The listing builds one solid part. Answer for the finished solid, in the listing's coordinates (mm). Coordinates: 2 decimals unless noted, no trailing zeros. Write each loop counter-clockwise with the first axis right and the second up, starting at its lowest first coordinate (ties: lowest second). Pieces come first, ordered by that corner, then holes.
from build123d import *

# Parameters (mm, degrees)
SKETCH1_W           = 203.2
SKETCH1_H           = 203.2
BASE_FLANGE1_DEPTH  = 1.5875
SKETCH6_R           = 1.5875
SKETCH6_R_2         = 2.413
SKETCH6_R_3         = 9.525
CUT_EXTRUDE1_DEPTH  = 288.372580731
BREAK_CORNER1_START = -1.5875
BREAK_CORNER1_DEPTH = 1.5875
SKETCH7_R           = 6.985
SKETCH7_R_2         = 13.97
SKETCH7_R_3         = 7.9375
SKETCH7_R_4         = 3.175
SKETCH7_R_5         = 2.159
CUT_EXTRUDE2_DEPTH  = 288.372580731


# Read off the part's stored shape, not the designer's step: Break-Corner1
# Sheet-metal steps are written as plain solids
with BuildPart() as part:
    # Sketch1 → Base-Flange1 (new body)
    with BuildSketch(Plane.XY):
        with Locations((101.6, 101.6)):
            Rectangle(SKETCH1_W, SKETCH1_H)
    extrude(amount=-BASE_FLANGE1_DEPTH)

    # Sketch6 → Cut-Extrude1 (cut, through all)
    with BuildSketch(Plane(origin=(0, 0, -1.5875), x_dir=(-1, 0, 0), z_dir=(0, 0, -1))):
        with Locations((-19.05, 139.7)):
            Circle(SKETCH6_R)
        with Locations((-19.05, 12.7)):
            Circle(SKETCH6_R)
        with Locations((-31.115, 48.768)):
            Circle(SKETCH6_R_2)
        with Locations((-31.115, 12.7)):
            Circle(SKETCH6_R_2)
        with Locations((-172.085, 48.768)):
            Circle(SKETCH6_R_2)
        with Locations((-172.085, 12.7)):
            Circle(SKETCH6_R_2)
        with Locations((-184.15, 139.7)):
            Circle(SKETCH6_R)
        with Locations((-184.15, 12.7)):
            Circle(SKETCH6_R)
        with Locations((-190.5, 38.1)):
            Circle(SKETCH6_R_3)
        with Locations((-190.5, 114.3)):
            Circle(SKETCH6_R_3)
        with Locations((-12.7, 114.3)):
            Circle(SKETCH6_R_3)
        with Locations((-12.7, 38.1)):
            Circle(SKETCH6_R_3)
        with Locations((-6.35, 76.2)):
            Circle(SKETCH6_R)
        with Locations((-196.85, 76.2)):
            Circle(SKETCH6_R)
    extrude(amount=-CUT_EXTRUDE1_DEPTH, mode=Mode.SUBTRACT)

    # Break-Corner1 outline → Break-Corner1 (cut)
    with BuildSketch(Plane.XY.offset(BREAK_CORNER1_START)):
        Polygon((0, 0), (3.175, 0), (0, 3.175), align=None)
        Polygon((203.2, 3.175), (200.025, 0), (203.2, 0), align=None)
        Polygon((0, 203.2), (0, 200.025), (3.175, 203.2), align=None)
        Polygon((200.025, 203.2), (203.2, 200.025), (203.2, 203.2), align=None)
    extrude(amount=BREAK_CORNER1_DEPTH, mode=Mode.SUBTRACT)

    # Sketch7 → Cut-Extrude2 (cut, through all)
    with BuildSketch(Plane(origin=(0, 0, -1.5875), x_dir=(-1, 0, 0), z_dir=(0, 0, -1))):
        with Locations((-177.8, 177.8)):
            Circle(SKETCH7_R)
        with Locations((-101.6, 177.8)):
            Circle(SKETCH7_R_2)
        with Locations((-25.4, 177.8)):
            Circle(SKETCH7_R)
        with Locations((-101.6, 114.3)):
            Circle(SKETCH7_R_3)
        with Locations((-112.7125, 93.218)):
            Circle(SKETCH7_R_4)
        with Locations((-90.4875, 93.218)):
            Circle(SKETCH7_R_4)
        with Locations((-130.556, 85.09)):
            Circle(SKETCH7_R_5)
        with Locations((-73.66, 67.31)):
            Circle(SKETCH7_R_5)
    extrude(amount=-CUT_EXTRUDE2_DEPTH, mode=Mode.SUBTRACT)


solid = part.part
1. Section C-C on z = -0.8 is taken. State how many separate pieces and enclosed holes the cut face has, then the cut area to 3 significant figures.
Results found:
separate pieces: 1
enclosed holes: 22
area: 38,800 mm2
2. Flat-ended cylindrical pins translate along their axes: P1, Ø10, axis at x = 24.5, y = 65.5, coming from the +Z side; P2, Ø3.5, axis at x = 130.556, y = 85.09, coming from the +Z side. Find the tip coordinate at first contact, or state that the pin passes through.
Results found:
P1: stops at z = 0
P2: passes through
3. Section B-B on y = 177.8 is taken. Give the vertices of the cut face in (x, z) (1 decimal).
Results found:
outline: (0, -1.6) - (18.4, -1.6) - (18.4, 0) - (0, 0) - close; (32.4, -1.6) - (87.6, -1.6) - (87.6, 0) - (32.4, 0) - close; (115.6, -1.6) - (170.8, -1.6) - (170.8, 0) - (115.6, 0) - close; (184.8, -1.6) - (203.2, -1.6) - (203.2, 0) - (184.8, 0) - close
4. Find the intervals of material crossed by L1, parallel to X at y = 139.7, z = -0.7; L2, parallel to Y at x = 190.5, z = -1.4 (3 decimals); L3, parallel to Y at x = 19.05, z = -0.7, in increasing order.
Results found:
L1: x = 0 to 17.46, 20.64 to 182.56, 185.74 to 203.2
L2: y = 0 to 28.575, 47.625 to 104.775, 123.825 to 203.2
L3: y = 0 to 11.11, 14.29 to 31, 45.2 to 107.2, 121.4 to 138.11, 141.29 to 174.89, 180.71 to 203.2
5. For a pull along X with two mould halves and no side action, classify faces 1 (the cylindrical face through (19.72, 120.74, -0.8)), 2 (the flat face through (100, 103, -1.588)) as pulls with the +X half, pulls with the -X half, needs draft (parallel to the pull), parting line crosses it, or undercut.
Results found:
face 1: undercut
face 2: needs draft
6. Section A-A on x = 25.4 is taken. Give the vertices of the cut face in (y, z) (1 decimal).
Results found:
outline: (0, -1.6) - (170.8, -1.6) - (170.8, 0) - (0, 0) - close; (184.8, -1.6) - (203.2, -1.6) - (203.2, 0) - (184.8, 0) - close
7. Section D-D on x = 112.5 is taken. Give the vertices of the cut face in (y, z).
Results found:
outline: (0, -1.59) - (90.05, -1.59) - (90.05, 0) - (0, 0) - close; (96.39, -1.59) - (169.06, -1.59) - (169.06, 0) - (96.39, 0) - close; (186.54, -1.59) - (203.2, -1.59) - (203.2, 0) - (186.54, 0) - close
